from build123d import *

# Parameters (mm, degrees)
F0_R     = 1.5
F1_DEPTH = 5


with BuildPart() as f1:
    # F0 (on Top) → F1 (new body)
    with BuildSketch(Plane.XY):
        with BuildLine():
            Line((-20.466092, 25.303127), (-10.897727, 25.303127))
            Line((-10.897727, 25.303127), (-10.897727, 23.303127))
            Line((-10.897727, 23.303127), (-18.466092, 23.303127))
            ThreePointArc((-18.466092, 23.303127), (-22.001626, 21.838661), (-23.466092, 18.303127))
            Line((-23.466092, 18.303127), (-23.466092, 15.104749))
            Line((-23.466092, 15.104749), (-23.466092, 9.20962))
            Line((-23.466092, 9.20962), (-23.466092, -4.459552))
            ThreePointArc((-23.466092, -4.459552), (-22.001626, -7.995086), (-18.466092, -9.459552))
            Line((-18.466092, -9.459552), (-5.325101, -9.459552))
            Line((-5.325101, -9.459552), (-5.325101, -3.459552))
            Line((-5.325101, -3.459552), (-12.466092, -3.459552))
            ThreePointArc((-12.466092, -3.459552), (-16.001626, -1.995086), (-17.466092, 1.540448))
            Line((-17.466092, 1.540448), (-17.466092, 13.303127))
            ThreePointArc((-17.466092, 13.303127), (-16.001626, 16.838661), (-12.466092, 18.303127))
            Line((-12.466092, 18.303127), (-5.325101, 18.303127))
            Line((-5.325101, 18.303127), (-5.325101, 23.303127))
            Line((-5.325101, 23.303127), (-3.195953, 23.303127))
            Line((-3.195953, 23.303127), (-3.195953, 18.303127))
            Line((-3.195953, 18.303127), (2.206437, 18.303127))
            Line((2.206437, 18.303127), (5.649895, 18.303127))
            ThreePointArc((5.649895, 18.303127), (9.185429, 16.838661), (10.649895, 13.303127))
            Line((10.649895, 13.303127), (10.649895, -1.416758))
            ThreePointArc((10.649895, -1.416758), (9.185429, -4.952292), (5.649895, -6.416758))
            Line((5.649895, -6.416758), (-3.195953, -6.416758))
            Line((-3.195953, -6.416758), (-3.195953, -12.416758))
            Line((-3.195953, -12.416758), (10.649895, -12.416758))
            Line((10.649895, -12.416758), (11.649895, -12.416758))
            ThreePointArc((11.649895, -12.416758), (15.185429, -10.952292), (16.649895, -7.416758))
            Line((16.649895, -7.416758), (16.649895, 18.303127))
            ThreePointArc((16.649895, 18.303127), (15.185429, 21.838661), (11.649895, 23.303127))
            Line((11.649895, 23.303127), (2.206437, 23.303127))
            Line((2.206437, 23.303127), (2.206437, 25.10515))
            Line((2.206437, 25.10515), (12.961418, 25.10515))
            ThreePointArc((12.961418, 25.10515), (14.626748, 24.869409), (16.161216, 24.180709))
            Line((16.161216, 24.180709), (18.022634, 23.00721))
            Line((18.022634, 23.00721), (20.078026, 24.866851))
            Line((20.078026, 24.866851), (17.85285, 26.679604))
            ThreePointArc((17.85285, 26.679604), (16.370805, 27.51388), (14.694856, 27.803127))
            Line((14.694856, 27.803127), (2.206437, 27.803127))
            Line((2.206437, 27.803127), (2.206437, 30.955919))
            Line((2.206437, 30.955919), (-3.195953, 30.955919))
            Line((-3.195953, 30.955919), (-3.195953, 25.303127))
            Line((-3.195953, 25.303127), (-5.295211, 25.303127))
            Line((-5.295211, 25.303127), (-5.295211, 30.303127))
            Line((-5.295211, 30.303127), (-31.466092, 30.303127))
            Line((-31.466092, 30.303127), (-31.466092, 26.543299))
            Line((-31.466092, 26.543299), (-31.466092, 6.599163))
            Line((-31.466092, 6.599163), (-25.466092, 6.599163))
            Line((-25.466092, 6.599163), (-25.466092, 20.303127))
            ThreePointArc((-25.466092, 20.303127), (-24.001626, 23.838661), (-20.466092, 25.303127))
        make_face()
        with Locations((-27.466092, 26.303127)):
            Circle(F0_R, mode=Mode.SUBTRACT)
    extrude(amount=F1_DEPTH)


solid = f1.part
Check sheet for the modelled part. Datum: model origin and axes. Units: mm. A direction names the side the tool comes from. Give positions to 0.01 mm unless a question says otherwise; leave off trailing zeros. Loops run counter-clockwise (first coordinate to the right, second up) from the corner with the lowest first, then second, coordinate; pieces in that order, holes last. Notation, with made-up numbers: M 77.5,77 L 94.5,77 A10 cw 94.5,89 Z; hole C -12.75,-35.5 d11. An arc over 180 degrees is marked long. Use a Markdown table: item, result. Add a question column.
Q1. Tool access check on faces 4 (the flat face through (-31.466, 19, 2)), 5 (the flat face through (2.206, 29, 2)), 6 (the flat face through (-5.325, -7, 2)), 7 (the flat face through (1, 18.303, 2)). Record the directions out of +Z, -Z, +X, -X, +Y, -Y that give a thin tool (end or side, any length) a straight path to the whole face; none if there is none.
Q2. Go/stop test with flat-tipped pins: pin 1 (2.5 mm diameter, centred on y = -5.5, z = 1.5, fed in from +X); pin 2 (2.5 mm diameter, centred on x = -16.5, z = 3, fed in from +Y); pin 3 (1.1 mm diameter, centred on x = -4, z = 3, fed in from -Y). Record where each tip stops, or that it passes through.
Q3. Sectioned sample at D-D, the plane x = 10. Record the cut outline in (y, z), then the cut area to 3 significant figures.
Q4. Sectioned sample at B-B, the plane y = 11.5. Record the cut outline in (x, z), then the cut area to 3 significant figures.
Q5. Sectioned sample at C-C, the plane y = 2.5. Record the cut outline in (x, z), then the cut area to 3 significant figures.
Q6. Scan lines: line 1 along X through (y, z) = (11, 1); line 2 along Y through (x, z) = (-6.5, 3.6); line 3 along X through (y, z) = (6, 2.6). Record each from-to range of solid material in increasing order. Write a range as [from, to].
Q7. Mould release check, pull along Y, two halves, no side actions. Record for faces 1 (the flat face through (9, 27.803, 2)), 2 (the flat face through (-12, -9.46, 2)), 3 (the cylindrical face through (-15.963, -2.034, 2.465)): pulls with the +Y half, pulls with the -Y half, needs draft (parallel to the pull), parting line crosses it, or undercut.
Q8. Sectioned sample at A-A, the plane x = -0.5. Record the cut outline in (y, z), then the cut area to 3 significant figures.
Verdict:
| question | item | result |
|---|---|---|
| 1 | face 4 | +Z, -Z, -X, +Y, -Y |
| 1 | face 5 | +Z, -Z, +X, +Y |
| 1 | face 6 | +Z, -Z, -Y |
| 1 | face 7 | +Z, -Z |
| 2 | pin 1 | x = 16.65 |
| 2 | pin 2 | y = 30.3 |
| 2 | pin 3 | y = 23.3 |
| 3 | outline | M -12.42,0 L -3.88,0 L -3.88,5 L -12.42,5 Z; M 15.77,0 L 23.3,0 L 23.3,5 L 15.77,5 Z; M 25.11,0 L 27.8,0 L 27.8,5 L 25.11,5 Z |
| 3 | area | 93.8 mm^2 |
| 4 | outline | M -31.47,0 L -25.47,0 L -25.47,5 L -31.47,5 Z; M -23.47,0 L -17.47,0 L -17.47,5 L -23.47,5 Z; M 10.65,0 L 16.65,0 L 16.65,5 L 10.65,5 Z |
| 4 | area | 90.0 mm^2 |
| 5 | outline | M -23.47,0 L -17.47,0 L -17.47,5 L -23.47,5 Z; M 10.65,0 L 16.65,0 L 16.65,5 L 10.65,5 Z |
| 5 | area | 60.0 mm^2 |
| 6 | line 1 | [-31.47, -25.47], [-23.47, -17.47], [10.65, 16.65] |
| 6 | line 2 | [-9.46, -3.46], [18.3, 30.3] |
| 6 | line 3 | [-23.47, -17.47], [10.65, 16.65] |
| 7 | face 1 | pulls with the +Y half |
| 7 | face 2 | pulls with the -Y half |
| 7 | face 3 | undercut |
| 8 | outline | M -12.42,0 L -6.42,0 L -6.42,5 L -12.42,5 Z; M 18.3,0 L 30.96,0 L 30.96,5 L 18.3,5 Z |
| 8 | area | 93.3 mm^2 |
